from build123d import *

# Parameters (mm, degrees)
PATTERN_CIRCULAR_1_COUNT = 6


with BuildPart() as part:
    # Эскиз1 → Повернуть1 (revolve)
    with BuildSketch(Plane(origin=(0, 0, 0), x_dir=(0, 0, -1), z_dir=(1, 0, 0))):
        Polygon((0, 26), (23, 26), (23, 19), (21, 19), (21, 21), (0, 21), align=None)
    revolve(axis=Axis((0, 0, 0), (0, 0, -1)))

    # Эскиз3 → Сверло под метчик  спиральное M2.51 (revolve, cut)
    with BuildSketch(Plane(origin=(23.5, 0, 0), x_dir=(0, -1, 0), z_dir=(1, 0, 0))):
        Polygon((0, 0), (0, 8.766097289), (1.275, 8), (1.275, 0), align=None)
    hole_wizard_m2_51 = revolve(axis=Axis((23.5, 0, 6.35), (0, 0, -1)), mode=Mode.SUBTRACT)

    # Круговой массив1: Сверло под метчик  спиральное M2.51 ×6 about axis
    pattern_circular_1_axis = Axis((0, 0, 0), (0, 0, 1))
    for i in range(1, PATTERN_CIRCULAR_1_COUNT):
        add(hole_wizard_m2_51.rotate(pattern_circular_1_axis, i * 360 / PATTERN_CIRCULAR_1_COUNT), mode=Mode.SUBTRACT)


solid = part.part
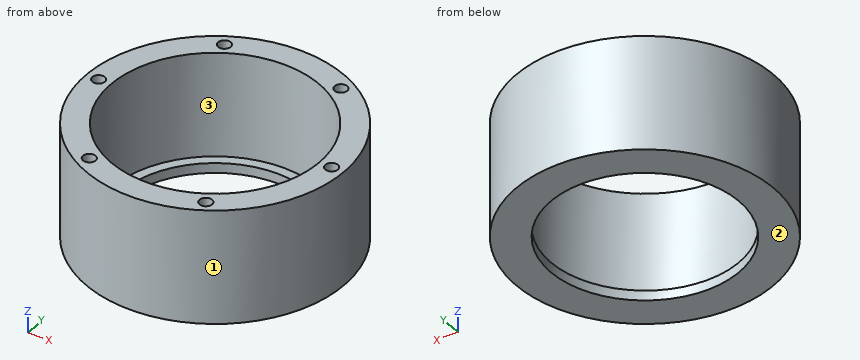
The listing builds one solid part. Answer for the finished solid, in the listing's coordinates (mm). Face numbers are marked on the shaded views. Round coordinates to 2 decimals unless told otherwise and drop trailing zeros. Order: outer loops, then holes, each group sorted by start corner. A loop starts at its lowest first (then second) coordinate and runs counter-clockwise, first axis right, second up. Notation, with made-up numbers: (3, -19) -> (58, -19) arc R17 ccw to (58, 13) -> close; hole circle Ø6 at (26, 6). An arc over 180 degrees is marked (long way). One line per item, written item: value.
Item 1: Find section B-B, the plane y = -11. Give the vertices of the cut face in (x, z).
Taken from the geometry:
outline: (-23.56, -23) -> (-15.49, -23) -> (-15.49, -21) -> (-17.89, -21) -> (-17.89, 0) -> (-23.56, 0) -> close; (15.49, -23) -> (23.56, -23) -> (23.56, 0) -> (17.89, 0) -> (17.89, -21) -> (15.49, -21) -> close
Item 2: Find section C-C, the plane z = -2.75. Give the vertices of the cut face in (x, y) (3 decimals), then the cut area to 3 significant figures.
Taken from the geometry:
outline: circle Ø52 at (0, 0); hole circle Ø2.55 at (-23.5, 0); hole circle Ø42 at (0, 0); hole circle Ø2.55 at (-11.75, -20.352); hole circle Ø2.55 at (-11.75, 20.352); hole circle Ø2.55 at (11.75, -20.352); hole circle Ø2.55 at (11.75, 20.352); hole circle Ø2.55 at (23.5, 0)
area: 708 mm2
Item 3: Given P1, Ø12, axis at x = -18.5, z = -19.5, coming from the -Y side; P2, Ø1, axis at x = 7.5, z = -7.5, coming from the -Y side; P3, Ø1, axis at x = -2.5, y = 16.5, coming from the -Z side; P4, Ø10, axis at y = 10, z = -6, coming from the -X side, each flat-ended and moving along its own axis, determine where each tip first touches the part or whether it passes through.
Taken from the geometry:
P1: stops at y = -22.8
P2: stops at y = -25.04
P3: passes through
P4: stops at x = -25.51
Item 4: Find section D-D, the plane z = -17.5. Give the vertices of the cut face in (x, y), then the cut area to 3 significant figures.
Taken from the geometry:
outline: circle Ø52 at (0, 0); hole circle Ø42 at (0, 0)
area: 738 mm2
Item 5: Straight lines are drawn through the part: L1, parallel to X at y = 0, z = -3 (3 decimals); L2, parallel to Z at x = -14, y = -14; L3, parallel to X at y = 5, z = -20.5. For each, find the intervals that lie inside material, in ascending order.
Taken from the geometry:
L1: x = -26 to -24.775, -22.225 to -21, 21 to 22.225, 24.775 to 26
L2: z = -23 to -21
L3: x = -25.51 to -20.4, 20.4 to 25.51
Item 6: Find section A-A, the plane x = -5.5. Give the vertices of the cut face in (y, z), then the cut area to 3 significant figures.
Taken from the geometry:
outline: (-25.41, -23) -> (-18.19, -23) -> (-18.19, -21) -> (-20.27, -21) -> (-20.27, 0) -> (-25.41, 0) -> close; (18.19, -23) -> (25.41, -23) -> (25.41, 0) -> (20.27, 0) -> (20.27, -21) -> (18.19, -21) -> close
area: 245 mm2
Item 7: For a pull along X with two mould halves and no side action, classify the marked faces 1, 2 and 3 as released by +X, released by -X, zero draft, split by the parting line, or undercut.
Taken from the geometry:
face 1: split by the parting line
face 2: zero draft
face 3: undercut
